Source: CAD feature listing. Evaluate the final solid. Frame: model axes, mm. A direction names the side the tool comes from. Give positions to 0.01 mm unless a question says otherwise; leave off trailing zeros. Write each loop counter-clockwise with the first axis right and the second up, starting at its lowest first coordinate (ties: lowest second). Pieces come first, ordered by that corner, then holes. Notation, with made-up numbers: (53.25, 39) - (76.25, 39) arc R26 ccw to (76.25, 58) - close; hole circle Ø6 at (-34.75, 26). An arc over 180 degrees is marked (long way). One line per question, with ' | ' between items. Start each with the question number.
(1) Access query for faces 1 (the flat face through (0, 3, 0)), 2 (the flat face through (0, -3, -2.5)). Directions: +Z, -Z, +X, -X, +Y, -Y. A direction counts if a zero-diameter tool reaches every point of the face in a straight line with its end or side. Return the directions, or none.
(2) Section A-A, the plane y = -2.25. Return loops of the section in (x, z), plus the area to 3 significant figures.
(3) Ray query, line 1 (X direction, y = -0.7, z = 0); line 2 (X direction, y = -1.05, z = 0); line 3 (X direction, y = 0.5, z = 5.5). Return the intervals inside material, ascending. Write a range as [from, to].
(4) Section C-C, the plane y = 1. State how many separate pieces and enclosed holes the cut face has, plus the area to 3 significant figures.
(5) Draft query along Z for faces 3 (the flat face through (0.6, -3, -2)), 4 (the flat face through (-4, -4, -9)), 5 (the cylindrical face through (9.98, -1.29, -0.66)), 6 (the flat face through (0, -3, 2.5)). Return one class per face: +Z half, -Z half, draft (parallel to the pull), parting line (faces both ways), or undercut.
(6) Section B-B, the plane z = 0. Return loops of the section in (x, y), plus the area to 3 significant figures.
(7) Pin query (flat end, axial travel): pin 1 (1 mm diameter, centred on y = -3.5, z = -3.5, fed in from -X); pin 2 (1.5 mm diameter, centred on x = -3, y = -1, fed in from -Z); pin 3 (1 mm diameter, centred on y = -2.5, z = 1.5, fed in from +X). Return the tip coordinate at first contact, or that it passes through.
```python
from build123d import *

# Parameters (mm, degrees)
SKETCH1_R           = 10
BOSS_EXTRUDE1_DEPTH = 3
SKETCH2_R           = 3
BOSS_EXTRUDE2_DEPTH = 5.5
FILLET1_R           = 0.5
CUT_EXTRUDE1_DEPTH  = 4.5
CHAMFER1_SIZE       = 1.5
CHAMFER1_SIZE2      = 0.866025404
CUT_EXTRUDE2_DEPTH  = 2
BOSS_EXTRUDE3_START = 4
SKETCH5_R           = 10
SKETCH5_R_2         = 8.5
BOSS_EXTRUDE3_DEPTH = 4
CHAMFER2_SIZE       = 1
FILLET2_R           = 0.5


with BuildPart() as part:
    # Sketch1 → Boss-Extrude1 (new body)
    with BuildSketch(Plane(origin=(0, 0, 0), x_dir=(1, 0, 0), z_dir=(0, 1, 0))):
        with Locations(Location((0, 0, 0), (0, 0, 270))):
            Circle(SKETCH1_R)
    extrude(amount=BOSS_EXTRUDE1_DEPTH)

    # Sketch2 → Boss-Extrude2 (add)
    with BuildSketch(Plane.XZ):
        with Locations(Location((0, 0, 0), (0, 0, 90))):
            Circle(SKETCH2_R)
    extrude(amount=BOSS_EXTRUDE2_DEPTH)

    # Fillet1
    fillet1_edges = [part.edges().sort_by_distance(p)[0] for p in [
        (0, 0, -3),
    ]]
    fillet(fillet1_edges, radius=FILLET1_R)

    # Sketch3 → Cut-Extrude1 (cut)
    with BuildSketch(Plane.XZ.offset(5.5)):
        Polygon((0.6, 0.6), (2.5, 0.6), (2.5, -0.6), (0.6, -0.6), (0.6, -2.5), (-0.6, -2.5), (-0.6, -0.6), (-2.5, -0.6), (-2.5, 0.6), (-0.6, 0.6), (-0.6, 2.5), (0.6, 2.5), align=None)
    extrude(amount=-CUT_EXTRUDE1_DEPTH, mode=Mode.SUBTRACT)

    # Chamfer1
    chamfer1_edges = [part.edges().sort_by_distance(p)[0] for p in [
        (0, 3, -10),
    ]]
    chamfer1_side = [part.faces().sort_by_distance(p)[0] for p in [
        (0, 1.5, -10),
    ]]
    chamfer(chamfer1_edges, length=CHAMFER1_SIZE, length2=CHAMFER1_SIZE2, reference=chamfer1_side[0])

    # Sketch4 → Cut-Extrude2 (cut)
    with BuildSketch(Plane.XZ):
        with BuildLine():
            Line((-0.785080982, 5.948112159), (-0.3672174, 5.548693088))
            add(Edge.make_bspline(
                [(-0.3672174, 5.548693088), (-0.331770807, 5.585344925), (-0.262532505, 5.656937445), (-0.150963545, 5.751719632), (-0.034935889, 5.830707761), (0.083293377, 5.89723106), (0.205850855, 5.947560676), (0.331319446, 5.984236716), (0.460500303, 6.006596711), (0.547924939, 6.00915509), (0.591897183, 6.010441886)],
                knots=[0, 0, 0, 0, 1.115251505, 2.178435587, 3.19620269, 4.182487026, 5.141301733, 6.088180966, 7.038406374, 8, 8, 8, 8], degree=3))
            add(Edge.make_bspline(
                [(0.591897183, 6.010441886), (0.62861935, 6.009425272), (0.701086501, 6.007419097), (0.807487269, 5.992711853), (0.909265103, 5.967701544), (1.006768403, 5.933232705), (1.099710263, 5.888631858), (1.188285547, 5.833933521), (1.272275875, 5.769631699), (1.350571785, 5.696059092), (1.422194132, 5.615675491), (1.485477036, 5.529906379), (1.538486619, 5.438948251), (1.581990722, 5.343722262), (1.615878736, 5.24378766), (1.640079036, 5.139211724), (1.654075842, 5.029869914), (1.65616496, 4.955540165), (1.65722671, 4.917763601)],
                knots=[0, 0, 0, 0, 1.035432265, 2.043311493, 3.022114605, 3.98653278, 4.95457646, 5.923598177, 6.917315552, 7.932509744, 8.948865224, 9.949768934, 10.933144597, 11.912367597, 12.897413939, 13.903909035, 14.934704909, 16, 16, 16, 16], degree=3))
            add(Edge.make_bspline(
                [(1.65722671, 4.917763601), (1.656920726, 4.891249365), (1.656317624, 4.83898926), (1.64971561, 4.761682062), (1.639084809, 4.686675803), (1.623699408, 4.614084098), (1.604459812, 4.543844039), (1.581887385, 4.475349668), (1.553570607, 4.409547423), (1.522138557, 4.345673054), (1.485583444, 4.285469453), (1.446170289, 4.228060322), (1.403433158, 4.173727077), (1.357095239, 4.122691832), (1.306504383, 4.075752155), (1.252968178, 4.031496513), (1.195583542, 3.991032776), (1.135542498, 3.95334546), (1.072326368, 3.920606168), (1.007650353, 3.890950695), (0.940533833, 3.866866041), (0.871793993, 3.847451613), (0.801676484, 3.830942542), (0.729495493, 3.820777399), (0.655876737, 3.813079455), (0.606122815, 3.812604152), (0.581084883, 3.812364963)],
                knots=[0, 0, 0, 0, 1.103660481, 2.175337485, 3.227646561, 4.255952547, 5.262355991, 6.258840057, 7.255597736, 8.242457506, 9.22035537, 10.185017736, 11.140346927, 12.096287581, 13.051739095, 14.01125915, 14.986044842, 15.97314143, 16.960198552, 17.947847494, 18.933482797, 19.925264591, 20.920966487, 21.929612487, 22.958107872, 24, 24, 24, 24], degree=3))
            add(Edge.make_bspline(
                [(0.581084883, 3.812364963), (0.53861625, 3.813593381), (0.455176427, 3.816006904), (0.332716491, 3.834880308), (0.216024371, 3.865925989), (0.122787926, 3.902589134), (0.049739634, 3.938794467), (-0.005870951, 3.972282616), (-0.06337663, 4.009742788), (-0.121822283, 4.05258877), (-0.181865308, 4.100306392), (-0.242445806, 4.153940761), (-0.30511465, 4.211725773), (-0.346168388, 4.252968071), (-0.3672174, 4.274113761)],
                knots=[0, 0, 0, 0, 1.404581149, 2.759636711, 4.088442092, 5.392261763, 6.066678138, 6.783632037, 7.538459478, 8.336747902, 9.180226004, 10.074962426, 11.012997595, 12, 12, 12, 12], degree=3))
            Line((-0.3672174, 4.274113761), (-0.772360629, 3.848617968))
            add(Edge.make_bspline(
                [(-0.772360629, 3.848617968), (-0.743881241, 3.821122013), (-0.688295566, 3.767455788), (-0.604446117, 3.691254757), (-0.520702197, 3.62277966), (-0.439086883, 3.55954515), (-0.358263232, 3.503393403), (-0.278239814, 3.454268339), (-0.19992253, 3.410927515), (-0.121685097, 3.374101852), (-0.04304068, 3.342833039), (0.037875183, 3.315912643), (0.12130986, 3.293138957), (0.207772931, 3.274763583), (0.296457921, 3.260029014), (0.388194805, 3.250083265), (0.482401925, 3.243397069), (0.546304074, 3.242796259), (0.578540813, 3.242493168)],
                knots=[0, 0, 0, 0, 1.244526981, 2.429050516, 3.560637417, 4.644440555, 5.67424972, 6.652764056, 7.595344123, 8.486817594, 9.369275933, 10.254498637, 11.166417451, 12.086725134, 13.032340136, 13.991389299, 14.986715468, 16, 16, 16, 16], degree=3))
            add(Edge.make_bspline(
                [(0.578540813, 3.242493168), (0.63775571, 3.244002674), (0.753622802, 3.246956357), (0.923423006, 3.26884115), (1.084728641, 3.305530621), (1.237932135, 3.357419651), (1.382984771, 3.423705456), (1.519849442, 3.504968741), (1.648305552, 3.6009936), (1.767315427, 3.710654531), (1.874965524, 3.831765824), (1.970115743, 3.961806126), (2.048824007, 4.101414539), (2.114177176, 4.248528599), (2.165282494, 4.403819647), (2.201251974, 4.567455659), (2.223434089, 4.739278634), (2.225860844, 4.856637687), (2.227098505, 4.916491566)],
                knots=[0, 0, 0, 0, 1.078019885, 2.10938526, 3.111377082, 4.085535484, 5.04941344, 6.010039228, 6.978205633, 7.964457913, 8.951525778, 9.924444315, 10.892603023, 11.863865945, 12.85144698, 13.863884204, 14.910567087, 16, 16, 16, 16], degree=3))
            add(Edge.make_bspline(
                [(2.227098505, 4.916491566), (2.22657553, 4.955527754), (2.22553912, 5.03288794), (2.21464636, 5.146845761), (2.199461218, 5.257934252), (2.175371372, 5.364999947), (2.146333439, 5.469485219), (2.110220954, 5.570254434), (2.067091593, 5.667597213), (2.018335518, 5.761676514), (1.963178258, 5.851876016), (1.901561543, 5.937420765), (1.835071629, 6.018971149), (1.76211087, 6.095445251), (1.683739482, 6.16751453), (1.599603627, 6.234788426), (1.510209341, 6.298231725), (1.415314666, 6.356208377), (1.316763153, 6.408651341), (1.215797795, 6.454908275), (1.112666654, 6.493568419), (1.007805777, 6.525635583), (0.900772127, 6.549571453), (0.792329685, 6.567690134), (0.681555734, 6.577818593), (0.607180623, 6.579476687), (0.569636566, 6.580313681)],
                knots=[0, 0, 0, 0, 1.071919942, 2.124283339, 3.142214191, 4.149696895, 5.136002878, 6.119640489, 7.086990633, 8.058538607, 9.028339693, 9.988281803, 10.952401235, 11.916291999, 12.888973767, 13.874849856, 14.873389453, 15.898127285, 16.927174885, 17.938320013, 18.946391617, 19.950418109, 20.947802303, 21.956882652, 22.968648068, 24, 24, 24, 24], degree=3))
            add(Edge.make_bspline(
                [(0.569636566, 6.580313681), (0.537607636, 6.579833895), (0.473882787, 6.578879311), (0.378985793, 6.570921817), (0.284847742, 6.558424654), (0.191805675, 6.539569095), (0.099194061, 6.517185164), (0.00822992, 6.487876495), (-0.082521756, 6.455206459), (-0.171637662, 6.416156102), (-0.259242191, 6.37352911), (-0.343283069, 6.32516724), (-0.425171333, 6.274046627), (-0.503092391, 6.217141729), (-0.578505869, 6.156516593), (-0.651017426, 6.091888368), (-0.71999073, 6.022179512), (-0.763274545, 5.97292609), (-0.785080982, 5.948112159)],
                knots=[0, 0, 0, 0, 0.996412454, 1.982464992, 2.961075852, 3.949442424, 4.934965278, 5.923860011, 6.921385422, 7.934793307, 8.949617135, 9.951082467, 10.950285876, 11.951772932, 12.951063433, 13.960125323, 14.972308753, 16, 16, 16, 16], degree=3))
        make_face()
        Polygon((-1.314247649, 6.580313681), (-1.884119443, 6.580313681), (-1.884119443, 5.644095732), (-2.250465597, 5.644095732), (-2.250465597, 5.155634194), (-1.884119443, 5.155634194), (-1.884119443, 3.323903425), (-1.314247649, 3.323903425), (-1.314247649, 5.155634194), (-1.029311751, 5.155634194), (-1.029311751, 5.644095732), (-1.314247649, 5.644095732), align=None)
    extrude(amount=-CUT_EXTRUDE2_DEPTH, mode=Mode.SUBTRACT)

    # Sketch5 → Boss-Extrude3 (add)
    with BuildSketch(Plane.XZ.offset(BOSS_EXTRUDE3_START)):
        with Locations(Location((0, 0, 0), (0, 0, 270))):
            Circle(SKETCH5_R)
        with Locations(Location((0, 0, 0), (0, 0, 270))):
            Circle(SKETCH5_R_2, mode=Mode.SUBTRACT)
    extrude(amount=-BOSS_EXTRUDE3_DEPTH)

    # Chamfer2
    chamfer2_edges = [part.edges().sort_by_distance(p)[0] for p in [
        (0, -4, 8.5),
    ]]
    chamfer(chamfer2_edges, length=CHAMFER2_SIZE)

    # Fillet2
    fillet2_edges = [part.edges().sort_by_distance(p)[0] for p in [
        (1.55, -5.5, -0.6),
        (1.55, -5.5, 0.6),
        (0.6, -5.5, 1.55),
        (-0.6, -5.5, 1.55),
        (-1.55, -5.5, 0.6),
        (-1.55, -5.5, -0.6),
        (-0.6, -5.5, -1.55),
        (0.6, -5.5, -1.55),
    ]]
    fillet(fillet2_edges, radius=FILLET2_R)


solid = part.part
```
Check sheet entries:
1) face 1: +Z, -Z, +X, -X, +Y | face 2: -Y
2) outline: circle Ø20 at (0, 0); circle Ø6 at (0, 0); hole circle Ø17 at (0, 0); hole (-2.5, -0.6) - (-0.6, -0.6) - (-0.6, -2.5) - (0.6, -2.5) - (0.6, -0.6) - (2.5, -0.6) - (2.5, 0.6) - (0.6, 0.6) - (0.6, 2.5) - (-0.6, 2.5) - (-0.6, 0.6) - (-2.5, 0.6) - close | area: 105 mm²
3) line 1: [-10, -8.5], [-3, 3], [8.5, 10] | line 2: [-10, -8.5], [-3, -2.5], [2.5, 3], [8.5, 10] | line 3: [-8.35, -2.25], [-1.03, 1.5], [2.13, 8.35]
4) separate pieces: 1 | enclosed holes: 2 | area: 308 mm²
5) face 3: undercut | face 4: draft | face 5: parting line | face 6: undercut
6) outline: (-10, -4) - (-9.5, -4) - (-8.5, -3) - (-8.5, 0) - (-3.5, 0) arc R0.5 cw to (-3, -0.5) - (-3, -5.5) - (-2.5, -5.5) - (-2.5, -1) - (2.5, -1) - (2.5, -5.5) - (3, -5.5) - (3, -0.5) arc R0.5 cw to (3.5, 0) - (8.5, 0) - (8.5, -3) - (9.5, -4) - (10, -4) - (10, 1.5) - (9.13, 3) - (-9.13, 3) - (-10, 1.5) - close | area: 80.3 mm²
7) pin 1: x = -9.54 | pin 2: z = -9.74 | pin 3: x = 9.95
